Autodesk Inventor part; units mm, degrees
ref_plane "YZ Plane" through (0, 0, 0) normal (1, 0, 0) x (0, 1, 0)
ref_plane "XZ Plane" through (0, 0, 0) normal (0, 1, 0) x (-1, 0, 0)
ref_plane "XY Plane" through (0, 0, 0) normal (0, 0, 1) x (1, 0, 0)
sketch "Эскиз1" plane through (0, 0, 0) normal (0, 0, 1) x (1, 0, 0)
  line L0 (-15.139, -15) -> (19.061, -15)
  line L1 (19.061, -15) -> (19.061, 10)
  line L2 (19.061, 10) -> (-15.139, 10)
  line L3 (-15.139, 10) -> (-15.139, -15)
  circle A0 centre (-11.139, 5) radius 1.6
  circle A1 centre (-11.139, -9) radius 1.6
  circle A2 centre (15.061, 5) radius 1.6
  circle A3 centre (15.061, -9) radius 1.6
  point P0 (0, 0)
  dimension "d0" = 34.2
  dimension "d5" = 3.2
  dimension "d7" = 14
  dimension "d16" = 3.2
  dimension "d17" = 3.2
  dimension "d18" = 3.2
  dimension "d19" = 5
  dimension "d20" = 14
  dimension "d21" = 6
  dimension "d22" = 6
  dimension "d23" = 4
  dimension "d24" = 4
extrude "Выдавливание1" add sketch "Эскиз1" along normal blind 2
chamfer "Фаска1" distance 4 angle 45 4 edges at (19.061, 10, 1) (-15.139, 10, 1) (19.061, -15, 1) (-15.139, -15, 1)
properties part number "стена_простая"
Can you work these out from the model? Positions are in its coordinate system, mm. Coordinates: 2 decimals unless noted, no trailing zeros. Loops run counter-clockwise (first coordinate to the right, second up) from the corner with the lowest first, then second, coordinate; pieces in that order, holes last. Notation, with made-up numbers: (38.25, 63.25) -> (61.25, 63.25) arc R17 ccw to (61.25, 90.25) -> close; hole circle Ø8 at (49.25, 45). An arc over 180 degrees is marked (long way). Answer as a JSON object with one key per item and string values.
1) Imagine slicing it at B-B (z = 0.45). Please give me the cut outline in (x, y), then the cut area to 3 significant figures.
Results:
{"outline": "(-15.14, -11) -> (-11.14, -15) -> (15.06, -15) -> (19.06, -11) -> (19.06, 6) -> (15.06, 10) -> (-11.14, 10) -> (-15.14, 6) -> close; hole circle Ø3.2 at (-11.14, -9); hole circle Ø3.2 at (-11.14, 5); hole circle Ø3.2 at (15.06, -9); hole circle Ø3.2 at (15.06, 5)", "area": "791 mm^2"}
2) For P1, Ø2.5, axis at x = -11.139, y = -9, coming from the +Z side, with a flat end and sliding along its axis, tell me the tip position at first contact or that it passes through.
Results:
{"P1": "passes through"}
3) Imagine slicing it at A-A (y = 5). Please give me the cut outline in (x, z).
Results:
{"outline": "(-15.14, 0) -> (-12.74, 0) -> (-12.74, 2) -> (-15.14, 2) -> close; (-9.54, 0) -> (13.46, 0) -> (13.46, 2) -> (-9.54, 2) -> close; (16.66, 0) -> (19.06, 0) -> (19.06, 2) -> (16.66, 2) -> close"}
4) If I drill on line 1 (Y direction, x = -11, z = 1.45); line 2 (Y direction, x = -12, z = 1.5); line 3 (X direction, y = 4, z = 1.2), over which ranges is the centre line in solid material (lowest first)?
Results:
{"line 1": "y = -15 to -10.59, -7.41 to 3.41, 6.59 to 10", "line 2": "y = -14.14 to -10.35, -7.65 to 3.65, 6.35 to 9.14", "line 3": "x = -15.14 to -12.39, -9.89 to 13.81, 16.31 to 19.06"}
5) Thinking about a two-plate mould opening in X: for faces 1 (the face through (-15.139, -2, 1)), 2 (the face through (16.54, -8.39, 0.99)), 3 (the face through (2, -15, 1)), which applies, pulls with the +X half, pulls with the -X half, needs draft (parallel to the pull), parting line crosses it, or undercut?
Results:
{"face 1": "pulls with the -X half", "face 2": "undercut", "face 3": "needs draft"}
